Geometry: final body of the model. Coordinates: model frame, mm. Round coordinates to 2 decimals unless told otherwise and drop trailing zeros. Write each loop counter-clockwise with the first axis right and the second up, starting at its lowest first coordinate (ties: lowest second). Pieces come first, ordered by that corner, then holes. Notation, with made-up numbers: (46, 66) -> (87, 66) arc R15 ccw to (87, 74) -> close; hole circle Ø10 at (76, 67). An arc over 180 degrees is marked (long way). Use one line per item in the form item = value. Start each with the question number.
1. Cut plane B-B, the plane z = 1.3. State how many separate pieces and enclosed holes the cut face has, plus the area to 3 significant figures.
2. Line query: L1, parallel to Y at x = -93, z = 1.3; L2, parallel to Y at x = 155, z = 0.85; L3, parallel to Y at x = 100, z = 0.35. Output: solid intervals per line, ascending.
3. Cut plane A-A, the plane x = -119.5. Return the cut outline in (y, z).
4. Cut plane C-C, the plane y = -134. Return the cut outline in (x, z).
5. Draft query along X for faces 1 (the face through (-131.426, 1.675, 0.811)), 2 (the face through (2, -2, 0)). Return one class per face: pulls with the +X half, pulls with the -X half, needs draft (parallel to the pull), parting line crosses it, or undercut.
6. Pin query (flat end, axial travel): pin 1 Ø0.8 at (x, z) = (134, 1) entering from -Y. Return the tip coordinate at first contact, or that it passes through.
7. Cut plane D-D, the plane x = 135. Return the cut outline in (y, z), plus the area to 3 significant figures.
```python
from build123d import *

# Parameters (mm, degrees)
BOSS_EXTRUDE1_DEPTH        = 1.6002
SKETCH2_R                  = 38.1
CUT_EXTRUDE1_DEPTH         = 2.6002
CIRPATTERN1_COUNT          = 8
F_10_CLEARANCE_HOLE1_D     = 5.1054
F_10_CLEARANCE_HOLE1_DEPTH = 129.53
F_10_CLEARANCE_HOLE1_TIP   = 1.533816902


with BuildPart() as part:
    # Sketch1 → Boss-Extrude1 (new body)
    with BuildSketch(Plane.XY):
        Polygon((161.3627, -22.34670835), (59.7625, -22.34670835), (59.7625, -153.41070835), (-161.3627, -153.41070835), (-161.3627, 145.48590835), (161.3627, 145.48590835), align=None)
    extrude(amount=BOSS_EXTRUDE1_DEPTH)

    # Sketch2 → Cut-Extrude1 (cut, through all)
    with BuildSketch(Plane.XY.offset(1.6002)):
        with Locations((-93.3627, 0)):
            Circle(SKETCH2_R)
    extrude(amount=-CUT_EXTRUDE1_DEPTH, mode=Mode.SUBTRACT)

    # Sketch11 → #4 Clearance Hole1 (revolve, cut)
    with BuildSketch(Plane(origin=(-93.3627, 50.8, 1.6002), x_dir=(0, -1, 0), z_dir=(1, 0, 0))):
        Polygon((0, 0), (0, 173.855187864), (1.4732, 172.97), (1.4732, 0), align=None)
    f_4_clearance_hole1 = revolve(axis=Axis((-93.3627, 50.8, 7.9502), (0, 0, -1)), mode=Mode.SUBTRACT)

    # CirPattern1: #4 Clearance Hole1 ×8 about axis
    cirpattern1_axis = Axis((-93.3627, 0, 0), (0, 0, 1))
    for i in range(1, CIRPATTERN1_COUNT):
        add(f_4_clearance_hole1.rotate(cirpattern1_axis, i * 360 / CIRPATTERN1_COUNT), mode=Mode.SUBTRACT)

    # #10 Clearance Hole1
    with Locations(Plane.XY.offset(1.6002)):
        with Locations((-155, 105.78570835), (155, 105.78570835), (-155, -105.78570835), (155, 25.27849165), (-155, 0)):
            Hole(F_10_CLEARANCE_HOLE1_D / 2, depth=F_10_CLEARANCE_HOLE1_DEPTH)
            with Locations((0, 0, -(F_10_CLEARANCE_HOLE1_DEPTH + F_10_CLEARANCE_HOLE1_TIP / 2))):  # 118° drill point
                Cone(0, F_10_CLEARANCE_HOLE1_D / 2, F_10_CLEARANCE_HOLE1_TIP, mode=Mode.SUBTRACT)


solid = part.part
```
Outcome:
q1.separate_pieces = 1
q1.enclosed_holes = 14
q1.area = 78,400 mm^2
q2.L1 = -153.41 to -52.23, -49.37 to -38.1, 38.1 to 49.37, 52.23 to 145.49
q2.L2 = -22.35 to 22.73, 27.83 to 103.23, 108.34 to 145.49
q2.L3 = -22.35 to 145.49
q3.outline = (-153.41, 0) -> (-27.72, 0) -> (-27.72, 1.6) -> (-153.41, 1.6) -> close; (27.72, 0) -> (145.49, 0) -> (145.49, 1.6) -> (27.72, 1.6) -> close
q4.outline = (-161.36, 0) -> (59.76, 0) -> (59.76, 1.6) -> (-161.36, 1.6) -> close
q5.face_1 = undercut
q5.face_2 = needs draft
q6.pin_1 = -22.35
q7.outline = (-22.35, 0) -> (145.49, 0) -> (145.49, 1.6) -> (-22.35, 1.6) -> close
q7.area = 269 mm^2
